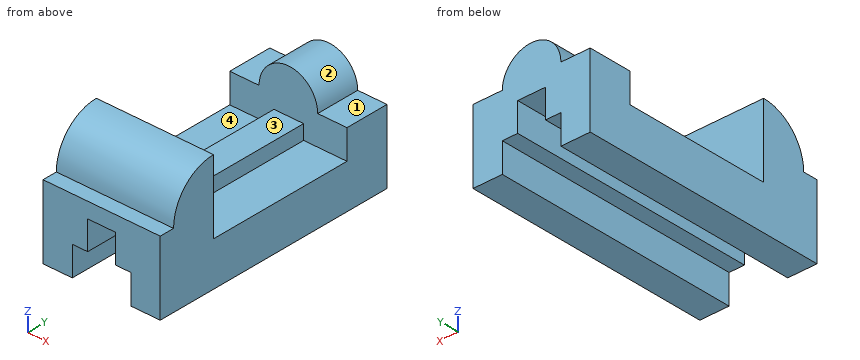
Autodesk Fusion 360 part; units mm, degrees
sketch "Sketch1" plane through (0, 0, 0) normal (0, 0, 1) x (1, 0, 0) in component "Component"
  line L0 (40, -85) -> (-40, -85)
  line L1 (-40, -85) -> (-40, 85)
  line L2 (-40, 85) -> (40, 85)
  line L3 (40, 85) -> (40, -85)
  line L4 (40, -85) -> (-40, 85) construction
  line L5 (-40, -85) -> (40, 85) construction
  dimension "d1" = 80
  dimension "d2" = 170
extrude "Extrude1" add sketch "Sketch1" along normal blind 30 in component "Component"
sketch "Sketch2" plane through (0, 0, 30) normal (0, 0, 1) x (-1, 0, 0) in component "Component"
  line L0 (-40, -85) -> (40, -85)
  line L1 (40, -85) -> (40, 85)
  line L2 (40, 85) -> (-40, 85)
  line L3 (-40, 85) -> (-40, -85)
  line L4 (40, 75) -> (-40, 75)
  dimension "d5" = 10
extrude "Extrude2" add sketch "Sketch2" along normal blind 20 contours L1 L2 L3 L4 in component "Component"
sketch "Sketch3" plane through (0, -85, 0) normal (0, -1, 0) x (1, 0, 0) in component "Component"
  line L0 (-40, 0) -> (40, 0)
  line L1 (40, 0) -> (40, 50)
  line L2 (40, 50) -> (-40, 50)
  line L3 (-40, 50) -> (-40, 0)
  line L4 (-20, 0) -> (-20, 20)
  line L5 (-20, 20) -> (-10, 20)
  line L6 (-10, 20) -> (-10, 40)
  line L7 (-10, 40) -> (10, 40)
  line L8 (10, 40) -> (10, 20)
  line L9 (10, 20) -> (20, 20)
  line L10 (20, 20) -> (20, 0)
sketch "Sketch4" plane through (0, 0, 30) normal (0, 0, 1) x (-1, 0, 0) in component "Component"
  line L0 (40, 75) -> (-40, 75)
  line L1 (-40, 75) -> (-40, -85)
  line L2 (-40, -85) -> (40, -85)
  line L3 (40, -85) -> (40, 75)
  line L4 (40, -55) -> (-40, -55)
  dimension "d10" = 30
extrude "Extrude4" add sketch "Sketch4" along normal blind 40 contours L1 L2 L3 L4 in component "Component"
sketch "Sketch5" plane through (0, 55, 0) normal (0, -1, 0) x (1, 0, 0) in component "Component"
  line L0 (-40, 30) -> (40, 30)
  line L1 (40, 30) -> (40, 70)
  line L2 (40, 70) -> (-40, 70)
  line L3 (-40, 70) -> (-40, 30)
  circle A0 centre (0, 50) radius 20
  line L4 (-40, 50) -> (40, 50)
  dimension "d13" = 40
  dimension "d14" = 20
extrude "Extrude5" cut sketch "Sketch5" against normal up to surface (30 mm away) contours L2 L3 A0 L4 | L1 L2 A0 L4 in component "Component"
sketch "Sketch6" plane through (0, 0, 30) normal (0, 0, 1) x (-1, 0, 0) in component "Component"
  line L0 (-40, -55) -> (40, -55)
  line L1 (40, -55) -> (40, 75)
  line L2 (40, 75) -> (-40, 75)
  line L3 (-40, 75) -> (-40, -55)
  line L4 (-40, 45) -> (40, 45)
  dimension "d17" = 30
extrude "Extrude6" add sketch "Sketch6" along normal blind 50 contours L1 L2 L3 L4 in component "Component"
sketch "Sketch7" plane through (40, 0, 0) normal (1, 0, 0) x (0, 1, 0) in component "Component"
  line L0 (85, 50) -> (55, 50)
  line L1 (55, 50) -> (55, 30)
  line L2 (55, 30) -> (-45, 30)
  line L3 (-45, 30) -> (-45, 80)
  line L4 (-45, 80) -> (-75, 80)
  line L5 (-75, 80) -> (-75, 50)
  line L6 (-75, 50) -> (-85, 50)
  line L7 (-85, 50) -> (-85, 0)
  line L8 (-85, 0) -> (85, 0)
  line L9 (85, 0) -> (85, 50)
  circle A0 centre (-45, 50) radius 30
  dimension "d20" = 60
extrude "Extrude7" cut sketch "Sketch7" against normal up to surface (80 mm away) contours L4 L5 A0 in component "Component"
sketch "Sketch8" plane through (0, -85, 0) normal (0, -1, 0) x (1, 0, 0) in component "Component"
  line L0 (-40, 0) -> (40, 0)
  line L1 (40, 0) -> (40, 50)
  line L2 (40, 50) -> (-40, 50)
  line L3 (-40, 50) -> (-40, 0)
  line L4 (-20, 0) -> (-20, 20)
  line L5 (-20, 20) -> (-10, 20)
  line L6 (10, 20) -> (20, 20)
  line L7 (20, 20) -> (20, 0)
  line L8 (10, 20) -> (-10, 20)
extrude "Extrude8" cut sketch "Sketch8" against normal up to surface (170 mm away) contours L0 L4 L5 L6 L7 L8 in component "Component"
sketch "Sketch10" plane through (0, 0, 30) normal (0, 0, 1) x (-1, 0, 0) in component "Component"
  line L0 (40, 45) -> (-40, 45)
  line L1 (-40, 45) -> (-40, -55)
  line L2 (-40, -55) -> (40, -55)
  line L3 (40, -55) -> (40, 45)
  line L4 (-10.4269, -55) -> (-10.4269, 45)
  line L5 (9.8376, 45) -> (9.8376, -55)
extrude "Extrude9" add sketch "Sketch10" along normal blind 10 contours L0 L2 L4 L5 in component "Component"
sketch "Sketch13" plane through (0, -85, 0) normal (0, -1, 0) x (1, 0, 0) in component "Component"
  line L0 (-20, 0) -> (-20, 20)
  line L1 (-20, 20) -> (20, 20)
  line L2 (20, 20) -> (20, 0)
  line L3 (20, 0) -> (40, 0)
  line L4 (40, 0) -> (40, 50)
  line L5 (40, 50) -> (-40, 50)
  line L6 (-40, 50) -> (-40, 0)
  line L7 (-40, 0) -> (-20, 0)
  line L8 (-10, 20) -> (-10, 40)
  line L9 (-10, 40) -> (10, 40)
  line L10 (10, 40) -> (10, 20)
  line L11 (-9.5, 20) -> (-9.5, 39.5)
  line L12 (-9.5, 39.5) -> (9.5, 39.5)
  line L13 (9.5, 39.5) -> (9.5, 20)
  dimension "d38" = 0.5
  dimension "d39" = 0.5
  dimension "d40" = 0.5
extrude "Extrude10" cut sketch "Sketch13" against normal up to surface (170 mm away) contours L1 L11 L12 L13 in component "Component"
component "Component" placed x (1, 0, 0) y (0, 1, 0) z (0, 0, 1) at (0, 0, 0)
Source: CAD feature listing. Evaluate the final solid. Frame: model axes, mm. Face numbers are marked on the shaded views. A direction names the side the tool comes from. Round coordinates to 2 decimals unless told otherwise and drop trailing zeros. Loops run counter-clockwise (first coordinate to the right, second up) from the corner with the lowest first, then second, coordinate; pieces in that order, holes last. Notation, with made-up numbers: M 6,80 L 57,80 A27 cw 57,101 Z; hole C 24.25,-15.5 d11. An arc over 180 degrees is marked long. Use a Markdown table: item, result. Add a question column.
1. Reachability of the marked faces 1, 2, 3 and 4 from +Z, -Z, +X, -X, +Y, -Y: full face, straight path, thin tool, end or side. Return the list, or none.
2. Section query C-C on y = -70.5. Return the cut outline in (x, z).
3. Section query B-B on x = 0. Return the cut outline in (y, z).
4. Section query A-A on z = 15. Return the cut outline in (x, y), then the cut area to 3 significant figures.
5. Line query: line 1 (X direction, y = -67.5, z = 18); line 2 (X direction, y = -51, z = 23); line 3 (Y direction, x = 16, z = 54.5). Output: solid intervals per line, ascending.
6. Section query D-D on z = 26. Return the cut outline in (x, y).
7. Contact query for flat-ended pins moving along their axis: P1, Ø4, axis at x = 25, z = 67, coming from the +Y side; P2, Ø11, axis at y = -18, z = 36, coming from the -X side; P3, Ø15, axis at x = 24, y = -4.5, coming from the +Z side. Output: stop coordinate, or through.
Reported:
| question | item | result |
|---|---|---|
| 1 | face 1 | +Z, +X, +Y |
| 1 | face 2 | +Z, +Y |
| 1 | face 3 | +Z, +X, -X |
| 1 | face 4 | +Z, -X |
| 2 | outline | M -40,0 L -20,0 L -20,20 L -9.5,20 L -9.5,39.5 L 9.5,39.5 L 9.5,20 L 20,20 L 20,0 L 40,0 L 40,65.8 L -40,65.8 Z |
| 3 | outline | M -85,39.5 L 85,39.5 L 85,70 L 55,70 L 55,40 L -45,40 L -45,80 A30 ccw -75,50 L -85,50 Z |
| 4 | outline | M -40,-85 L -20,-85 L -20,85 L -40,85 Z; M 20,-85 L 40,-85 L 40,85 L 20,85 Z |
| 4 | area | 6,800 mm² |
| 5 | line 1 | x = -40 to -20, 20 to 40 |
| 5 | line 2 | x = -40 to -9.5, 9.5 to 40 |
| 5 | line 3 | y = -74.66 to -45, 55 to 85 |
| 6 | outline | M -40,-85 L -9.5,-85 L -9.5,85 L -40,85 Z; M 9.5,-85 L 40,-85 L 40,85 L 9.5,85 Z |
| 7 | P1 | stops at y = -45 |
| 7 | P2 | stops at x = -9.84 |
| 7 | P3 | stops at z = 30 |
